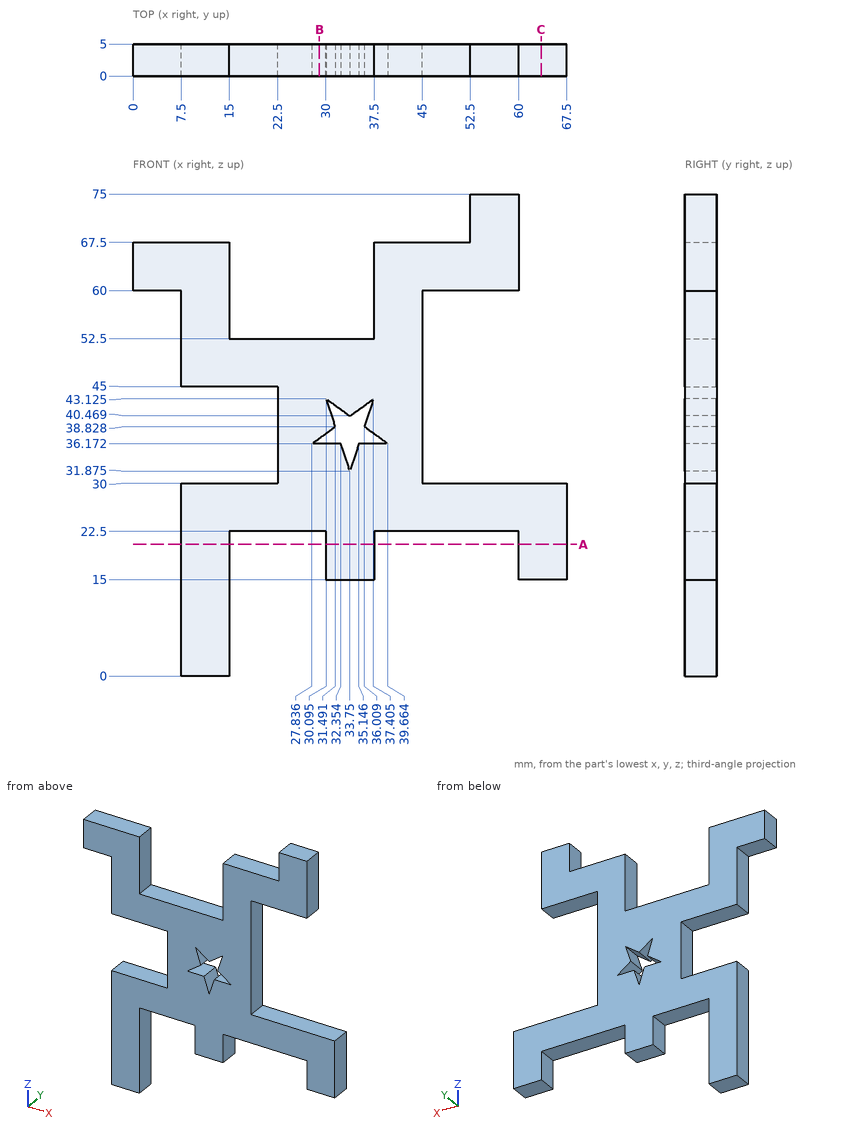
Job drawing, mm, ordinate dimensions from the low corner. One solid piece. Coordinates: 2 decimals unless noted, no trailing zeros. Order: outer loops, then holes, each group sorted by start corner. A loop starts at its lowest first (then second) coordinate and runs counter-clockwise, first axis right, second up. Notation, with made-up numbers: (12.25, 66) -> (20.25, 66) arc R22 cw to (20.25, 89) -> close; hole circle Ø2 at (85, 41). An arc over 180 degrees is marked (long way). Return JSON: item names as keys, results as strings. Group by question number.
Item 1: Saw through at B-B on x = 29. Write the cut outline in (y, z).
Item 2: Saw through at C-C on x = 63.5. Write the cut outline in (y, z).
Item 3: Saw through at A-A on z = 20.5. Write the cut outline in (x, y).
Item 4: Wall check: line 1 along Z through (x, y) = (10, 0.3); line 2 along Z through (x, y) = (55.5, 0.55); line 3 along X through (y, z) = (3.5, 63). Give the ranges that are in metal, low to high. Write a range as [from, to].
Item 5: Flat gauge pins, fed straight in: P1, Ø1.5, axis at y = 2.5, z = 20, coming from the -X side; P2, Ø1.5, axis at x = 42, y = 3.5, coming from the +Z side; P3, Ø1.5, axis at y = 1.5, z = 37, coming from the -X side. Where does each tip first touch, or does it go through?
Values found:
{
 "1": {"outline": "(0, 22.5) -> (5, 22.5) -> (5, 36.17) -> (0, 36.17) -> close; (0, 37.02) -> (5, 37.02) -> (5, 52.5) -> (0, 52.5) -> close"},
 "2": {"outline": "(0, 15) -> (5, 15) -> (5, 30) -> (0, 30) -> close"},
 "3": {"outline": "(7.5, 0) -> (15, 0) -> (15, 5) -> (7.5, 5) -> close; (30, 0) -> (37.5, 0) -> (37.5, 5) -> (30, 5) -> close; (60, 0) -> (67.5, 0) -> (67.5, 5) -> (60, 5) -> close"},
 "4": {"line 1": "z = [0, 30], [45, 67.5]", "line 2": "z = [22.5, 30], [60, 75]", "line 3": "x = [0, 15], [37.5, 60]"},
 "5": {"P1": "stops at x = 7.5", "P2": "stops at z = 67.5", "P3": "stops at x = 22.5"}
}
